```python
from build123d import *

# Parameters (mm, degrees)
Y_KSEKLIK_EKSTR_ZYON1_DEPTH = 3
Y_KSEKLIK_EKSTR_ZYON2_DEPTH = 3
Y_KSEKLIK_EKSTR_ZYON3_DEPTH = 3
Y_KSEKLIK_EKSTR_ZYON4_DEPTH = 41
M3_BO_LUKLU_DELIK1_D        = 3.2
M3_BO_LUKLU_DELIK1_DEPTH    = 10
M3_BO_LUKLU_DELIK1_TIP      = 0.96137699
IZIM10_W                    = 25.3
IZIM10_H                    = 25.3
KES_EKSTR_ZYON1_DEPTH       = 10


with BuildPart() as part:
    # izim1 → Y_kseklik-Ekstr_zyon1 (new body)
    with BuildSketch(Plane.XY):
        Polygon((67, 0), (0, 0), (0, 80), (10, 80), (10, 50), (57, 50), (57, 80), (67, 80), align=None)
    extrude(amount=Y_KSEKLIK_EKSTR_ZYON1_DEPTH)

    # izim4 → Y_kseklik-Ekstr_zyon3 (add)
    with BuildSketch(Plane.ZY.offset(-57)):
        Polygon((3, 80), (-23.280562552, 80), (-23.280562552, 69.037921865), (0, 45.757359313), (3, 45.757359313), align=None)
    extrude(amount=Y_KSEKLIK_EKSTR_ZYON3_DEPTH)



with BuildPart() as body_2:
    # izim2 → Y_kseklik-Ekstr_zyon2 (new body)
    with BuildSketch(Plane(origin=(10, 0, 0), x_dir=(0, 0, -1), z_dir=(1, 0, 0))):
        Polygon((-3, 80), (23.280562552, 80), (23.280562552, 69.037921865), (0, 45.757359313), (-3, 45.757359313), align=None)
    extrude(amount=Y_KSEKLIK_EKSTR_ZYON2_DEPTH)


with BuildPart() as part_1:
    add(part.part)

    add(body_2.part)  # Y_kseklik-Ekstr_zyon4 merges body 2
    # izim5 → Y_kseklik-Ekstr_zyon4 (add)
    with BuildSketch(Plane.ZY.offset(-54)):
        Polygon((0, 45.757359313), (-23.280562552, 69.037921865), (-23.280562552, 80), (-20.280562552, 80), (-20.280562552, 70.280562552), (0, 50), align=None)
    extrude(amount=Y_KSEKLIK_EKSTR_ZYON4_DEPTH)

    # M3 Bo_luklu Delik1
    with Locations(Plane.XY.offset(3)):
        with Locations((62.25, 60), (33.5, 15), (4.75, 60)):
            Hole(M3_BO_LUKLU_DELIK1_D / 2, depth=M3_BO_LUKLU_DELIK1_DEPTH)
            with Locations((0, 0, -(M3_BO_LUKLU_DELIK1_DEPTH + M3_BO_LUKLU_DELIK1_TIP / 2))):  # 118° drill point
                Cone(0, M3_BO_LUKLU_DELIK1_D / 2, M3_BO_LUKLU_DELIK1_TIP, mode=Mode.SUBTRACT)

    # izim10 → Kes-Ekstr_zyon1 (cut)
    with BuildSketch(Plane(origin=(0, 22.878679656, 22.878679656), x_dir=(1, 0, 0), z_dir=(0, -0.7071067811865438, -0.7071067811865513))):
        with Locations((33.5, -48.77902636)):
            Rectangle(IZIM10_W, IZIM10_H)
    extrude(amount=-KES_EKSTR_ZYON1_DEPTH, mode=Mode.SUBTRACT)


solid = part_1.part
```
The model under review builds one solid part; all positions refer to its coordinate system, in mm. A direction names the side the tool comes from. Round coordinates to 2 decimals unless told otherwise and drop trailing zeros. Order: outer loops, then holes, each group sorted by start corner. A loop starts at its lowest first (then second) coordinate and runs counter-clockwise, first axis right, second up.
(1) Take a section at A-A, the plane x = 45. State the section outline as (y, z) points.
Working result:
outline: (0, 0) - (45.76, 0) - (48.43, -2.67) - (50.55, -0.55) - (50, 0) - (50, 3) - (0, 3) - close; (66.32, -20.56) - (69.04, -23.28) - (80, -23.28) - (80, -20.28) - (70.28, -20.28) - (68.44, -18.44) - close
(2) Take a section at B-B, the plane y = 63.5. State the section outline as (x, z) points.
Working result:
outline: (0, 0) - (10, 0) - (10, -17.74) - (20.85, -17.74) - (20.85, -13.5) - (13, -13.5) - (13, 3) - (0, 3) - close; (46.15, -17.74) - (57, -17.74) - (57, 0) - (67, 0) - (67, 3) - (54, 3) - (54, -13.5) - (46.15, -13.5) - close
(3) Mouldability with a two-part tool opening along X and no side actions: class faces 1 (the face through (0, 39, 1)), 2 (the face through (33, 80, -21)), 3 (the face through (20.85, 59, -11)), 4 (the face through (33.323, 67.361, -19.512)) as released by +X, released by -X, zero draft, split by the parting line, or undercut.
Working result:
face 1: released by -X
face 2: zero draft
face 3: undercut
face 4: undercut
(4) Wall thickness on L1, parallel to Y at x = 62.25, z = 2.2; L2, parallel to Y at x = 33.5, z = 0.75; L3, parallel to Z at x = 25, y = 12.5: over which ranges is each line inside the solid? List them lowest first.
Working result:
L1: y = 0 to 58.4, 61.6 to 80
L2: y = 0 to 13.4, 16.6 to 50
L3: z = 0 to 3
(5) Tool access review of faces 5 (the face through (34.68, 16.08, 1.48)), 6 (the face through (57, 67, -9)), 7 (the face through (33.323, 49.472, -1.623)), 8 (the face through (34, 75, -20.281)): name each direction out of +Z, -Z, +X, -X, +Y, -Y from which nothing blocks a thin tool from reaching the whole face with its end or side.
Working result:
face 5: +Z, -Z
face 6: -Z, +X, +Y, -Y
face 7: -Z, +Y
face 8: +Z, +Y
(6) For P1, Ø10.5, axis at x = 39, y = 77, coming from the +Z side; P2, Ø3, axis at x = 25.5, z = -18.5, coming from the +Y side; P3, Ø6, axis at y = 63, z = -10.5, coming from the -X side, all flat-tipped, find the tip position at first contact; note any pin that passes through.
Working result:
P1: stops at z = -20.28
P2: stops at y = 70
P3: stops at x = 10
(7) Take a section at C-C, the plane x = 33.5. State the section outline as (y, z) points.
Working result:
outline: (0, 0) - (13.4, 0) - (13.4, 3) - (0, 3) - close; (16.6, 0) - (45.76, 0) - (48.43, -2.67) - (50.55, -0.55) - (50, 0) - (50, 3) - (16.6, 3) - close; (66.32, -20.56) - (69.04, -23.28) - (80, -23.28) - (80, -20.28) - (70.28, -20.28) - (68.44, -18.44) - close
(8) Take a section at D-D, the plane z = -9. State the section outline as (x, y) points, plus the area to 3 significant figures.
Working result:
outline: (10, 54.76) - (20.85, 54.76) - (20.85, 59) - (13, 59) - (13, 80) - (10, 80) - close; (46.15, 54.76) - (57, 54.76) - (57, 80) - (54, 80) - (54, 59) - (46.15, 59) - close
area: 218 mm2
